```python
from build123d import *

# Parameters (mm, degrees)
F0_W     = 100
F0_H     = 40
F1_DEPTH = 5
F2_R     = 10
F2_R_2   = 2.5
F3_DEPTH = 5
F4_W     = 5
F4_H     = 5
F5_DEPTH = 5


with BuildPart() as f1:
    # F0 (on Front) → F1 (new body)
    with BuildSketch(Plane.XZ):
        Rectangle(F0_W, F0_H)
    extrude(amount=F1_DEPTH)

    # F2 (on face) → F3 (cut, through all)
    with BuildSketch(Plane.XZ.offset(5)):
        with Locations((-33, 0)):
            Circle(F2_R)
        Circle(F2_R_2)
        with Locations((33, 0)):
            Circle(F2_R)
    extrude(amount=-F3_DEPTH, mode=Mode.SUBTRACT)

    # F4 (on face) → F5 (cut, through all)
    with BuildSketch(Plane.XZ.offset(5)):
        with Locations((0, 17.5)):
            Rectangle(F4_W, F4_H)
    extrude(amount=-F5_DEPTH, mode=Mode.SUBTRACT)


solid = f1.part
```
Here's how the part is built. I have some questions about the finished solid (model axes, mm). A direction names the side the tool comes from. Coordinates: 2 decimals unless noted, no trailing zeros. Loops run counter-clockwise (first coordinate to the right, second up) from the corner with the lowest first, then second, coordinate; pieces in that order, holes last. Notation, with made-up numbers: (-8.75, 75.5) - (26.25, 75.5) arc R32 ccw to (26.25, 112.5) - close; hole circle Ø1 at (28, 44). An arc over 180 degrees is marked (long way). Answer as CSV lines item,"result".
Q1. If I drill on L1, parallel to X at y = -2.4, z = 15.5; L2, parallel to X at y = -3.3, z = 7.5; L3, parallel to Z at x = 33, y = -2.75, over which ranges is the centre line in solid material (lowest first)? Write a range as [from, to].
Response:
L1,"[-50, -2.5], [2.5, 50]"
L2,"[-50, -39.61], [-26.39, 26.39], [39.61, 50]"
L3,"[-20, -10], [10, 20]"
Q2. If we section it at B-B, the plane z = 17.5: Write out the boundary of the cut face in (x, y), and give its area (3 significant figures).
Response:
outline,"(-50, -5) - (-2.5, -5) - (-2.5, 0) - (-50, 0) - close; (2.5, -5) - (50, -5) - (50, 0) - (2.5, 0) - close"
area,"475 mm2"
Q3. For faces 5 (the face through (-2.5, -3, 17)), 6 (the face through (-1, 0, -4)), which set-ups out of +Z, -Z, +X, -X, +Y, -Y let a thin tool reach every point of the face, with its end or its side?
Response:
face 5,"+Z, +Y, -Y"
face 6,"+Z, -Z, +X, -X, +Y"
Q4. We'd pull the mould along Z, two halves only. Please class faces 1 (the face through (-27, -2, 20)), 2 (the face through (2.5, -3, 17)), 3 (the face through (-0.54, -2.54, -2.44)), 4 (the face through (-1, -2, -20)): pulls with the +Z half, pulls with the -Z half, needs draft (parallel to the pull), parting line crosses it, or undercut.
Response:
face 1,"pulls with the +Z half"
face 2,"needs draft"
face 3,"undercut"
face 4,"pulls with the -Z half"
Q5. If we section it at D-D, the plane y = -3.6: Write out the boundary of the cut face in (x, z), and give its area (3 significant figures).
Response:
outline,"(-50, -20) - (50, -20) - (50, 20) - (2.5, 20) - (2.5, 15) - (-2.5, 15) - (-2.5, 20) - (-50, 20) - close; hole circle Ø20 at (-33, 0); hole circle Ø5 at (0, 0); hole circle Ø20 at (33, 0)"
area,"3,330 mm2"
Q6. If we section it at A-A, the plane z = 0: Write out the boundary of the cut face in (x, y).
Response:
outline,"(-50, -5) - (-43, -5) - (-43, 0) - (-50, 0) - close; (-23, -5) - (-2.5, -5) - (-2.5, 0) - (-23, 0) - close; (2.5, -5) - (23, -5) - (23, 0) - (2.5, 0) - close; (43, -5) - (50, -5) - (50, 0) - (43, 0) - close"
Q7. If we section it at C-C, the plane x = 0: Write out the boundary of the cut face in (y, z).
Response:
outline,"(-5, -20) - (0, -20) - (0, -2.5) - (-5, -2.5) - close; (-5, 2.5) - (0, 2.5) - (0, 15) - (-5, 15) - close"
